from build123d import *

# Parameters (mm, degrees)
SKETCH_1_R      = 2.75
SKETCH_1_R_2    = 2.423316248
EXTRUDE_1_DEPTH = 3


with BuildPart() as part:
    # 草图1 → 凸台-拉伸1 (new body)
    with BuildSketch(Plane(origin=(0, 0, 0), x_dir=(1, 0, 0), z_dir=(0, 1, 0))):
        with BuildLine():
            Line((-6, 48), (6, 48))
            ThreePointArc((6, 48), (7.414213562, 47.414213562), (8, 46))
            Line((8, 46), (8, 10))
            ThreePointArc((8, 10), (8.585786438, 8.585786438), (10, 8))
            Line((10, 8), (19.538252224, 8))
            ThreePointArc((19.538252224, 8), (20.952465786, 7.414213562), (21.538252224, 6))
            Line((21.538252224, 6), (21.538252224, -6))
            ThreePointArc((21.538252224, -6), (20.952465786, -7.414213562), (19.538252224, -8))
            Line((19.538252224, -8), (10, -8))
            ThreePointArc((10, -8), (8.585786438, -8.585786438), (8, -10))
            Line((8, -10), (8, -46))
            ThreePointArc((8, -46), (7.414213562, -47.414213562), (6, -48))
            Line((6, -48), (-6, -48))
            ThreePointArc((-6, -48), (-7.414213562, -47.414213562), (-8, -46))
            Line((-8, -46), (-8, -10))
            ThreePointArc((-8, -10), (-8.585786438, -8.585786438), (-10, -8))
            Line((-10, -8), (-19.538252224, -8))
            ThreePointArc((-19.538252224, -8), (-20.952465786, -7.414213562), (-21.538252224, -6))
            Line((-21.538252224, -6), (-21.538252224, 6))
            ThreePointArc((-21.538252224, 6), (-20.952465786, 7.414213562), (-19.538252224, 8))
            Line((-19.538252224, 8), (-10, 8))
            ThreePointArc((-10, 8), (-8.585786438, 8.585786438), (-8, 10))
            Line((-8, 10), (-8, 46))
            ThreePointArc((-8, 46), (-7.414213562, 47.414213562), (-6, 48))
        make_face()
        with Locations(Location((0, 38, 0), (0, 0, 270))):
            Circle(SKETCH_1_R, mode=Mode.SUBTRACT)
        with Locations(Location((0, 16, 0), (0, 0, 270))):
            Circle(SKETCH_1_R, mode=Mode.SUBTRACT)
        with Locations(Location((0, -16, 0), (0, 0, 90))):
            Circle(SKETCH_1_R, mode=Mode.SUBTRACT)
        with Locations(Location((0, -38, 0), (0, 0, 90))):
            Circle(SKETCH_1_R, mode=Mode.SUBTRACT)
        with Locations(Location((-15.538252224, 0, 0), (0, 0, 270))):
            Circle(SKETCH_1_R_2, mode=Mode.SUBTRACT)
        with Locations(Location((15.538252224, 0, 0), (0, 0, 90))):
            Circle(SKETCH_1_R_2, mode=Mode.SUBTRACT)
    extrude(amount=EXTRUDE_1_DEPTH)


solid = part.part
Could you check a few things on this model? Use its own coordinates, in mm. A direction names the side the tool comes from. Round coordinates to 2 decimals unless told otherwise and drop trailing zeros. Write each loop counter-clockwise with the first axis right and the second up, starting at its lowest first coordinate (ties: lowest second). Pieces come first, ordered by that corner, then holes. Notation, with made-up numbers: (15.25, 22.25) -> (66.25, 22.25) arc R20 cw to (66.25, 51.25) -> close; hole circle Ø6 at (64.25, -9). An arc over 180 degrees is marked (long way). Use a Markdown table: item, result.
1. For pin 1 Ø7 at (x, z) = (0, 38) entering from +Y; pin 2 Ø1.5 at (y, z) = (1.5, 24.5) entering from +X; pin 3 Ø1.5 at (x, y) = (-16, 1) entering from -Z; pin 4 Ø1.5 at (x, y) = (-16.5, 1.5) entering from +Z, each with a flat end and sliding along its axis, tell me the tip position at first contact or that it passes through.
Answer key:
| item | result |
|---|---|
| pin 1 | stops at y = 3 |
| pin 2 | stops at x = 8 |
| pin 3 | stops at z = -8 |
| pin 4 | stops at z = 8 |
2. If we section it at B-B (z = 0): List the corners of the cut face in (x, y) for me.
Answer key:
| item | result |
|---|---|
| outline | (-21.54, 0) -> (-17.96, 0) -> (-17.96, 3) -> (-21.54, 3) -> close; (-13.11, 0) -> (13.11, 0) -> (13.11, 3) -> (-13.11, 3) -> close; (17.96, 0) -> (21.54, 0) -> (21.54, 3) -> (17.96, 3) -> close |
3. Which directions (+Z, -Z, +X, -X, +Y, -Y) give clear straight access to the entire face, cutting with the end or side of a thin tool? Please do faces 1 (the face through (-15, 1, 8)), 2 (the face through (8, 1, 28)), 3 (the face through (8, 1, -28)).
Answer key:
| item | result |
|---|---|
| face 1 | +Z, -X, +Y, -Y |
| face 2 | +Z, +X, +Y, -Y |
| face 3 | -Z, +X, +Y, -Y |
4. We'd pull the mould along Z, two halves only. Please class faces 4 (the face through (7.43, 1.48, 47.4)), 5 (the face through (-15, 1, -8)), 6 (the face through (-17.904, 1.479, -0.525)), 7 (the face through (-0.121, 1.479, 40.747)): +Z half, -Z half, draft (parallel to the pull), parting line (faces both ways), or undercut.
Answer key:
| item | result |
|---|---|
| face 4 | +Z half |
| face 5 | -Z half |
| face 6 | undercut |
| face 7 | undercut |
5. If we section it at A-A (x = 0): List the corners of the cut face in (y, z) for me.
Answer key:
| item | result |
|---|---|
| outline | (0, -48) -> (3, -48) -> (3, -40.75) -> (0, -40.75) -> close; (0, -35.25) -> (3, -35.25) -> (3, -18.75) -> (0, -18.75) -> close; (0, -13.25) -> (3, -13.25) -> (3, 13.25) -> (0, 13.25) -> close; (0, 18.75) -> (3, 18.75) -> (3, 35.25) -> (0, 35.25) -> close; (0, 40.75) -> (3, 40.75) -> (3, 48) -> (0, 48) -> close |
6. If we section it at C-C (z = -16): List the corners of the cut face in (x, y) for me.
Answer key:
| item | result |
|---|---|
| outline | (-8, 0) -> (-2.75, 0) -> (-2.75, 3) -> (-8, 3) -> close; (2.75, 0) -> (8, 0) -> (8, 3) -> (2.75, 3) -> close |
7. If we section it at D-D (y = 1.2): State how many separate pieces and enclosed holes the cut face has, then the cut area to 3 significant figures.
Answer key:
| item | result |
|---|---|
| separate pieces | 1 |
| enclosed holes | 6 |
| area | 1,830 mm^2 |
8. Please list where these lines run through material, in increasing order: probe 1 along X at (y, z) = (1.45, 0); probe 2 along X at (y, z) = (2.3, -16); probe 3 along Z at (x, y) = (-10, 1.75).
Answer key:
| item | result |
|---|---|
| probe 1 | x = -21.54 to -17.96, -13.11 to 13.11, 17.96 to 21.54 |
| probe 2 | x = -8 to -2.75, 2.75 to 8 |
| probe 3 | z = -8 to 8 |
